```python
from build123d import *

# Parameters (mm, degrees)
F0_R      = 9.5
F1_DEPTH  = 5
F2_R      = 1
F4_R      = 3
F6_R      = 2
F8_R      = 2.6
F9_DEPTH  = 3
F10_DEPTH = 5
F11_SIZE  = 0.5


with BuildPart() as f1:
    # F0 (on Top) → F1 (new body)
    with BuildSketch(Plane.XY):
        Circle(F0_R)
    extrude(amount=F1_DEPTH)

    # F2
    f2_edges = [f1.edges().sort_by_distance(p)[0] for p in [
        (-9.5, 0, 0),
    ]]
    fillet(f2_edges, radius=F2_R)



with BuildPart() as f7:
    # F4 (on offset) → F7 section 0
    with BuildSketch(Plane.XY.offset(8)):
        Circle(F4_R)
    # F6 (on offset) → F7 section 1
    with BuildSketch(Plane.XY.offset(12)):
        Circle(F6_R)
    loft()


with BuildPart() as f1_1:
    add(f1.part)

    add(f7.part)  # F9 merges F7
    # F8 (on face) → F9 (join)
    with BuildSketch(Plane.XY.offset(5)):
        Circle(F8_R)
    extrude(amount=F9_DEPTH)

    # F10 (add): a face of the model
    f10_faces = [f1_1.faces().sort_by_distance(p)[0] for p in [
        (0, 0, 12),
    ]]
    extrude(f10_faces, amount=F10_DEPTH)

    # F11
    f11_edges = [f1_1.edges().sort_by_distance(p)[0] for p in [
        (-2, 0, 17),
    ]]
    chamfer(f11_edges, length=F11_SIZE)


solid = f1_1.part
```
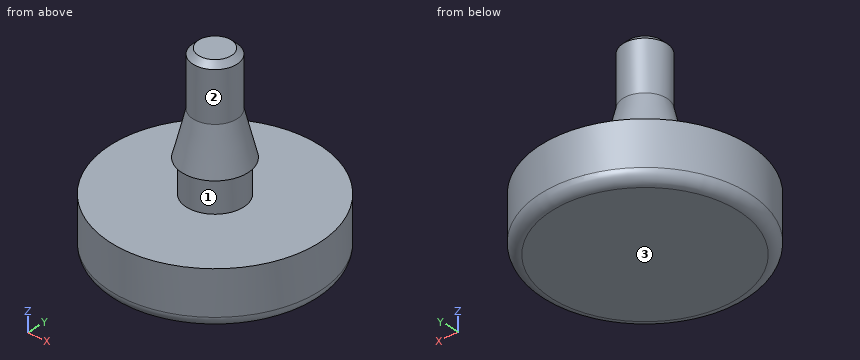
Design review of the part built by this model. Coordinates are the model's own, in mm. Face numbers are marked on the shaded views. Round coordinates to 2 decimals unless told otherwise and drop trailing zeros. Order: outer loops, then holes, each group sorted by start corner. A loop starts at its lowest first (then second) coordinate and runs counter-clockwise, first axis right, second up. Notation, with made-up numbers: (43, 70) - (50, 70) arc R18 ccw to (50, 97) - close; hole circle Ø11 at (43, 62). An arc over 180 degrees is marked (long way). Return JSON: item names as keys, results as strings.
Q1. For pin 1 Ø3 at (x, y) = (4, 7) entering from +Z; pin 2 Ø1.5 at (x, z) = (1, 9.5) entering from -Y; pin 3 Ø1.5 at (y, z) = (0, 12) entering from -X, all flat-tipped, find the tip position at first contact; note any pin that passes through.
Computed values:
{"pin 1": "stops at z = 5", "pin 2": "stops at y = -2.72", "pin 3": "stops at x = -2.19"}
Q2. Wall thickness on L1, parallel to Z at x = -6.25, y = 4.25; L2, parallel to Y at x = 1.5, z = 4.75; L3, parallel to Y at x = -6.5, z = 1.25: over which ranges is each line inside the solid? List them lowest first. Write a range as [from, to].
Computed values:
{"L1": "z = [0, 5]", "L2": "y = [-9.38, 9.38]", "L3": "y = [-6.93, 6.93]"}
Q3. The part is to be moulded in two halves that separate along Z. For the marked faces 1, 2 and 3, say which applies: pulls with the +Z half, pulls with the -Z half, needs draft (parallel to the pull), parting line crosses it, or undercut.
Computed values:
{"face 1": "undercut", "face 2": "needs draft", "face 3": "pulls with the -Z half"}
Q4. Consider section A-A on x = 0. Write out the cut boundary in (y, z).
Computed values:
{"outline": "(-9.5, 1) arc R1 ccw to (-8.5, 0) - (8.5, 0) arc R1 ccw to (9.5, 1) - (9.5, 5) - (2.6, 5) - (2.6, 8) - (3, 8) - (2, 12) - (2, 16.5) - (1.5, 17) - (-1.5, 17) - (-2, 16.5) - (-2, 12) - (-3, 8) - (-2.6, 8) - (-2.6, 5) - (-9.5, 5) - close"}
Q5. Consider section B-B on z = 15.75. Write out the cut boundary in (x, y), plus the area to 3 significant figures.
Computed values:
{"outline": "circle Ø4 at (0, 0)", "area": "12.6 mm2"}
Q6. Consider section C-C on z = 2.75. Write out the cut boundary in (x, y).
Computed values:
{"outline": "circle Ø19 at (0, 0)"}
